from build123d import *

# Parameters (mm, degrees)
F1_DEPTH = 19.05
F2_R     = 3.175
F3_DEPTH = 35.561
F4_R     = 3.175
F5_DEPTH = 19.05


with BuildPart() as f1:
    # F0 (on Front) → F1 (new body)
    with BuildSketch(Plane.XZ):
        Polygon((-30.315266, 20.453066), (-41.745266, 20.453066), (-41.745266, -17.646934), (-6.185266, -17.646934), (-6.185266, 20.453066), (-17.615266, 20.453066), (-17.615266, -1.620747), (-30.315266, -1.620747), align=None)
    extrude(amount=F1_DEPTH)

    # F2 (on face) → F3 (cut, through all)
    with BuildSketch(Plane.YZ.offset(-6.185266)):
        with Locations((-9.525, 7.753066)):
            Circle(F2_R)
    extrude(amount=-F3_DEPTH, mode=Mode.SUBTRACT)

    # F4 (on face) → F5 (cut)
    with BuildSketch(Plane(origin=(0, 0, -17.646934), x_dir=(1, 0, 0), z_dir=(0, 0, -1))):
        with Locations((-36.970066, 12.7)):
            Circle(F4_R)
        with Locations((-10.960466, 12.7)):
            Circle(F4_R)
    extrude(amount=-F5_DEPTH, mode=Mode.SUBTRACT)


solid = f1.part
Input: part model. Units: mm. Frame: model coordinates. A direction names the side the tool comes from. Give positions to 0.01 mm unless a question says otherwise; leave off trailing zeros. Write each loop counter-clockwise with the first axis right and the second up, starting at its lowest first coordinate (ties: lowest second). Pieces come first, ordered by that corner, then holes. Notation, with made-up numbers: (-23, 10.25) -> (-7, 10.25) arc R16 cw to (-7, 38.25) -> close; hole circle Ø3 at (81, 57.5). An arc over 180 degrees is marked (long way). Use one line per item in the form item = value. Start each with the question number.
1) Set-up query: faces 5 (the cylindrical face through (-13.48, -10.77, -8.26)), 6 (the flat face through (-24, -9, -1.621)), 7 (the cylindrical face through (-35.95, -9.94, 10.9)). Return all of +Z, -Z, +X, -X, +Y, -Y with unobstructed straight access to the full face (end or side cutting, diameter ignored); none if empty.
2) Pin query (flat end, axial travel): pin 1 (1.9 mm diameter, centred on x = -11, y = -12, fed in from -Z); pin 2 (10 mm diameter, centred on x = -23.5, y = -12.5, fed in from +Z). Return the tip coordinate at first contact, or that it passes through.
3) Section query C-C on y = -2. Return the cut outline in (x, z), then the cut area to 3 significant figures.
4) Ray query, probe 1 along X at (y, z) = (-2.75, 15.5); probe 2 along X at (y, z) = (-12.7, -3.25); probe 3 along X at (y, z) = (-15.5, -13.5). Return the intervals inside material, ascending. Write a range as from..to.
5) Section query A-A on z = -14.5. Return the cut outline in (x, y) (3 decimals).
6) Section query B-B on x = -9. Return the cut outline in (y, z) (3 decimals).
7) Draft query along Y for faces 1 (the flat face through (-37, -13, 1.403)), 2 (the flat face through (-24, 0, -3)), 3 (the flat face through (-24, -19.05, -3)), 4 (the flat face through (-6.185, -9, 1)). Return one class per face: pulls with the +Y half, pulls with the -Y half, needs draft (parallel to the pull), parting line crosses it, or undercut.
8) Section query D-D on y = -10.75. Return the cut outline in (x, z), then the cut area to 3 significant figures.
Outcome:
q1.face_5 = -Z
q1.face_6 = +Z, +Y, -Y
q1.face_7 = +X, -X
q2.pin_1 = 1.4
q2.pin_2 = -1.62
q3.outline = (-41.75, -17.65) -> (-6.19, -17.65) -> (-6.19, 20.45) -> (-17.62, 20.45) -> (-17.62, -1.62) -> (-30.32, -1.62) -> (-30.32, 20.45) -> (-41.75, 20.45) -> close
q3.area = 1,070 mm^2
q4.probe_1 = -41.75..-30.32, -17.62..-6.19
q4.probe_2 = -41.75..-40.15, -33.8..-14.14, -7.79..-6.19
q4.probe_3 = -41.75..-38.47, -35.47..-12.46, -9.46..-6.19
q5.outline = (-41.745, -19.05) -> (-6.185, -19.05) -> (-6.185, 0) -> (-41.745, 0) -> close; hole circle Ø6.35 at (-36.97, -12.7); hole circle Ø6.35 at (-10.96, -12.7)
q6.outline = (-19.05, -17.647) -> (-15.197, -17.647) -> (-15.197, 1.403) -> (-10.203, 1.403) -> (-10.203, -17.647) -> (0, -17.647) -> (0, 20.453) -> (-19.05, 20.453) -> close; hole circle Ø6.35 at (-9.525, 7.753)
q7.face_1 = undercut
q7.face_2 = pulls with the +Y half
q7.face_3 = pulls with the -Y half
q7.face_4 = needs draft
q8.outline = (-41.75, -17.65) -> (-39.48, -17.65) -> (-39.48, 1.4) -> (-34.46, 1.4) -> (-34.46, -17.65) -> (-13.47, -17.65) -> (-13.47, 1.4) -> (-8.45, 1.4) -> (-8.45, -17.65) -> (-6.19, -17.65) -> (-6.19, 4.82) -> (-17.62, 4.82) -> (-17.62, -1.62) -> (-30.32, -1.62) -> (-30.32, 4.82) -> (-41.75, 4.82) -> close; (-41.75, 10.68) -> (-30.32, 10.68) -> (-30.32, 20.45) -> (-41.75, 20.45) -> close; (-17.62, 10.68) -> (-6.19, 10.68) -> (-6.19, 20.45) -> (-17.62, 20.45) -> close
q8.area = 750 mm^2
